The drawing under review shows one solid part. Ordinate dimensions are in mm from its lowest x, y, z. Give positions to 0.01 mm unless a question says otherwise; leave off trailing zeros. Loops run counter-clockwise (first coordinate to the right, second up) from the corner with the lowest first, then second, coordinate; pieces in that order, holes last. Notation, with made-up numbers: M 8.25,85.5 L 26.25,85.5 A13 cw 26.25,99.5 Z; hole C 51.25,-23 d6. An arc over 180 degrees is marked long. Answer as CSV lines item,"result".
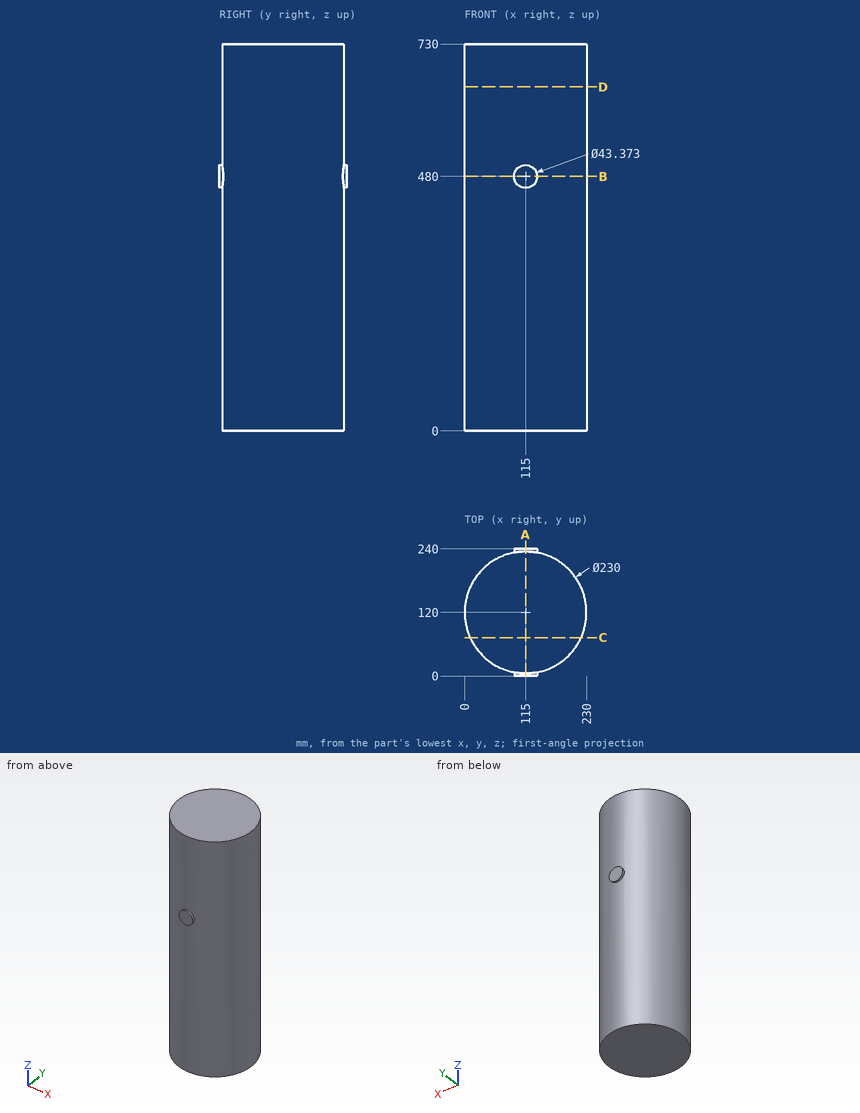
1. For P1, Ø5, axis at y = 83.5, z = 287, coming from the +X side; P2, Ø8, axis at y = 78, z = 189.5, coming from the -X side; P3, Ø5, axis at x = 180, y = 216, coming from the +Z side; P4, Ø10, axis at y = 130.5, z = 493, coming from the -X side, all flat-tipped, find the tip position at first contact; note any pin that passes through.
Answer block:
P1,"x = 224.86"
P2,"x = 6.46"
P3,"z = 730"
P4,"x = 0.13"
2. We need section C-C, the plane y = 72.5. Write out the cut boundary in (x, z), plus the area to 3 significant figures.
Answer block:
outline,"M 10.27,0 L 219.73,0 L 219.73,730 L 10.27,730 Z"
area,"153,000 mm²"
3. We need section B-B, the plane z = 480. Write out the cut boundary in (x, y), plus the area to 3 significant figures.
Answer block:
outline,"M 93.31,0 L 136.69,0 L 136.69,7.06 A115 ccw 136.69,232.94 L 136.69,240 L 93.31,240 L 93.31,232.94 A115 ccw 93.31,7.06 Z"
area,"42,000 mm²"
4. We need section A-A, the plane x = 115. Write out the cut boundary in (y, z).
Answer block:
outline,"M 0,458.31 L 5,458.31 L 5,0 L 235,0 L 235,458.31 L 240,458.31 L 240,501.69 L 235,501.69 L 235,730 L 5,730 L 5,501.69 L 0,501.69 Z"
5. To check wall thickness, follow L1, parallel to X at y = 115.5, z = 386.5; L2, parallel to X at y = 184.5, z = 690.5; L3, parallel to Y at x = 15, z = 426. State the ranges of each line that lie inside material, in increasing order. Write a range as [from, to].
Answer block:
L1,"[0.09, 229.91]"
L2,"[19.79, 210.21]"
L3,"[63.21, 176.79]"
6. We need section D-D, the plane z = 649. Write out the cut boundary in (x, y), plus the area to 3 significant figures.
Answer block:
outline,"C 115,120 d230"
area,"41,500 mm²"
